Model file for the job. Use its own axes, mm. A direction names the side the tool comes from. Round coordinates to 2 decimals unless told otherwise and drop trailing zeros. Order: outer loops, then holes, each group sorted by start corner. A loop starts at its lowest first (then second) coordinate and runs counter-clockwise, first axis right, second up. Notation, with made-up numbers: M 85.5,43.5 L 111.5,43.5 A25 ccw 111.5,64.5 Z; hole C 49.5,-7.75 d1. An arc over 180 degrees is marked long. Return JSON: item names as keys, results as strings. Group by question number.
Item 1: Pin check, flat tips, straight feed: pin 1 Ø5.5 at (x, z) = (34.925, 0) entering from +Y; pin 2 Ø2 at (y, z) = (-3, 4.5) entering from -X; pin 3 Ø3 at (y, z) = (-4, 6.5) entering from -X; pin 4 Ø1 at (x, z) = (-6.5, -7.5) entering from -Y. Stop position of each tip, or through.
Item 2: Slice it at B-B on y = -2.5. Give the number of separate pieces and of enclosed holes in the cut face, then the cut area to 3 significant figures.
Item 3: Pull direction Z, two halves, no side cores. Call faces 1 (the face through (-10, -3, 9.525)), 2 (the face through (39.468, -3.131, 1.431)), 3 (the face through (-39.683, -3.131, 0.209)), 4 (the face through (-42.787, -3.219, -5.377)): pulls with the +Z half, pulls with the -Z half, needs draft (parallel to the pull), parting line crosses it, or undercut.
Item 4: Slice it at D-D on z = -3. Write the cut outline in (x, y), then the cut area to 3 significant figures.
Item 5: Probe line 1 along X through (y, z) = (-5, 0.25); line 2 along X through (y, z) = (-0.75, 1.5); line 3 along Z through (x, y) = (-38, -1.5). List the from-to ranges inside material, lowest first.
Item 6: Slice it at A-A on z = 2.75. Write the cut outline in (x, y), then the cut area to 3 significant figures.
Item 7: Which spindle directions (+Z, -Z, +X, -X, +Y, -Y) get a long thin tool onto all of the face, cutting with end or side? Do faces 5 (the face through (-11, -4.762, -8)), 6 (the face through (-11, -1.588, 8)), 7 (the face through (-11, -1.588, -8)), 8 (the face through (9, -1, -6.35)), 9 (the face through (-11, -4.762, 8)). Say none if no direction does.
from build123d import *

# Parameters (mm, degrees)
F0_R          = 4.7625
F1_DEPTH      = 6.35
F5_DEPTH      = 1.5875
F5_DEPTH_BACK = 1.5875
F6_SIZE       = 3.17499
F7_R          = 9.52499


# Not quite as in the source:
# - a fillet or chamfer is up to 0.001 mm smaller than in the source, because OpenCascade refuses the exact size


with BuildPart() as f1:
    # F0 (on Front) → F1 (new body)
    with BuildSketch(Plane.XZ):
        with BuildLine():
            ThreePointArc((44.45, 3.81), (43.7060512242, 5.6060512242), (41.91, 6.35))
            Line((41.91, 6.35), (-41.91, 6.35))
            ThreePointArc((-41.91, 6.35), (-43.7060512242, 5.6060512242), (-44.45, 3.81))
            Line((-44.45, 3.81), (-44.45, -3.81))
            ThreePointArc((-44.45, -3.81), (-43.7060512242, -5.6060512242), (-41.91, -6.35))
            Line((-41.91, -6.35), (41.91, -6.35))
            ThreePointArc((41.91, -6.35), (43.7060512242, -5.6060512242), (44.45, -3.81))
            Line((44.45, -3.81), (44.45, 3.81))
        make_face()
        with Locations((-34.925, 0)):
            Circle(F0_R, mode=Mode.SUBTRACT)
        with Locations((34.925, 0)):
            Circle(F0_R, mode=Mode.SUBTRACT)
    extrude(amount=F1_DEPTH)

    # F4 (on face) → F5 (join, two sides)
    with BuildSketch(Plane(origin=(0, -3.175, 0), x_dir=(-1, 0, 0), z_dir=(0, 1, 0))) as f5_sk:
        Polygon((36.3781489432, 5.461), (44.45, 0), (44.45, 9.525), (-19.05, 9.525), (-19.05, 5.461), (29.7344345599, 5.461), align=None)
        Polygon((-19.05, -5.461), (-19.05, -9.525), (44.45, -9.525), (44.45, 0), (36.3781489432, -5.461), (29.7344345599, -5.461), align=None)
    extrude(amount=F5_DEPTH)
    extrude(f5_sk.sketch, amount=-F5_DEPTH_BACK)

    # F6 (size 3.175 in the source; OpenCascade refuses exactly that, so slightly less here)
    f6_edges = [f1.edges().sort_by_distance(p)[0] for p in [
        (19.05, -3.175, 9.525),
        (19.05, -3.175, -9.525),
    ]]
    chamfer(f6_edges, length=F6_SIZE)

    # F7 (radius 9.525 in the source; OpenCascade refuses exactly that, so slightly less here)
    f7_edges = [f1.edges().sort_by_distance(p)[0] for p in [
        (-44.45, -3.175, 9.525),
        (-44.45, -3.175, -9.525),
    ]]
    fillet(f7_edges, radius=F7_R)


solid = f1.part
Output values:
{
 "1": {"pin 1": "through", "pin 2": "x = -43.78", "pin 3": "x = -43.03", "pin 4": "y = -4.76"},
 "2": {"separate pieces": "1", "enclosed holes": "2", "area": "1,340 mm²"},
 "3": {"face 1": "pulls with the +Z half", "face 2": "undercut", "face 3": "undercut", "face 4": "pulls with the -Z half"},
 "4": {"outline": "M -43.97,-6.35 L -38.62,-6.35 L -38.62,0 L -43.97,0 Z; M -31.23,-6.35 L 31.23,-6.35 L 31.23,0 L -31.23,0 Z; M 38.62,-6.35 L 44.45,-6.35 L 44.45,0 L 38.62,0 Z", "area": "467 mm²"},
 "5": {"line 1": "-44.45 to -39.68, -30.17 to 30.17, 39.68 to 44.45", "line 2": "-44.33 to -39.45, -30.4 to 30.4, 39.45 to 44.45", "line 3": "-6.35 to -3.64, 3.64 to 6.35"},
 "6": {"outline": "M -44.04,-6.35 L -38.81,-6.35 L -38.81,0 L -44.04,0 Z; M -31.04,-6.35 L 31.04,-6.35 L 31.04,0 L -31.04,0 Z; M 38.81,-6.35 L 44.45,-6.35 L 44.45,0 L 38.81,0 Z", "area": "463 mm²"},
 "7": {"face 5": "-Z, +X, -X, -Y", "face 6": "+Z, +X, -X, +Y", "face 7": "-Z, +X, -X, +Y", "face 8": "-Z, +X", "face 9": "+Z, +X, -X, -Y"}
}
